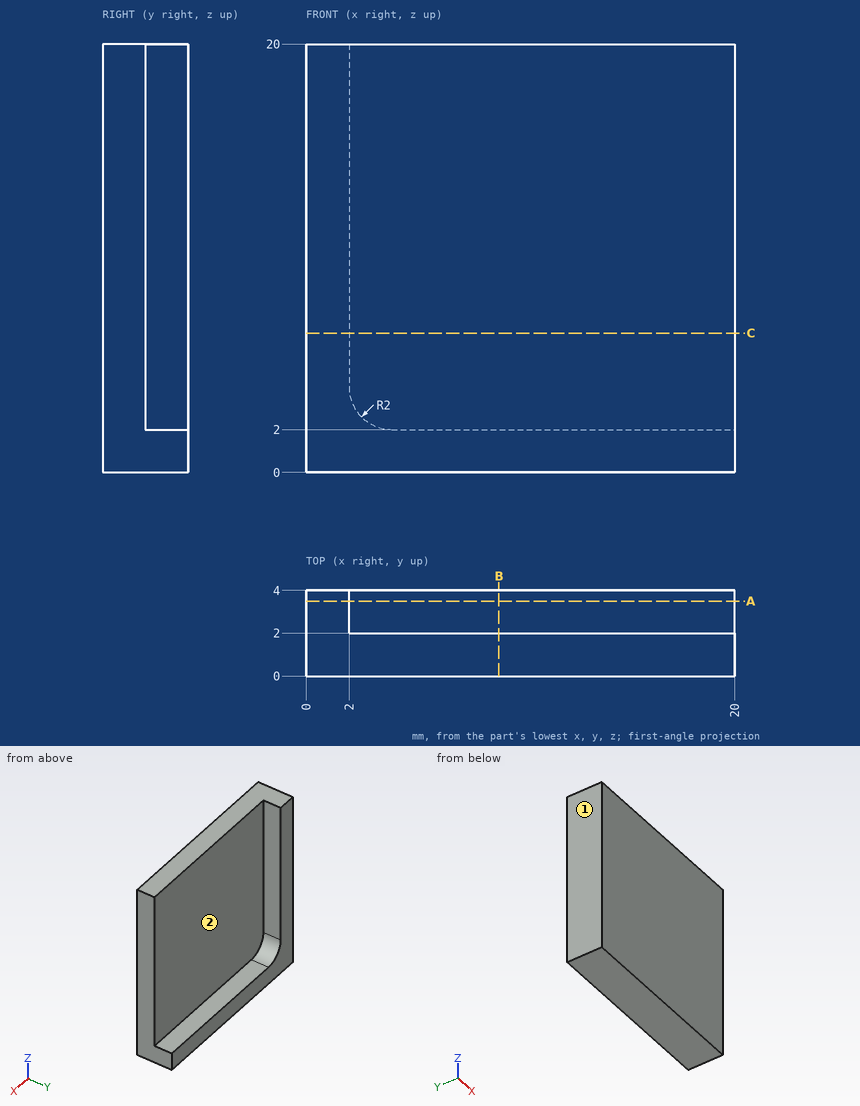
Can you work these out from the drawing? Everything is in mm from the part's minimum corner. A direction names the side the tool comes from. Round coordinates to 2 decimals unless told otherwise and drop trailing zeros. Loops run counter-clockwise (first coordinate to the right, second up) from the corner with the lowest first, then second, coordinate; pieces in that order, holes last. Notation, with made-up numbers: M -18.5,26 L -9.5,26 A16 cw -9.5,43 Z; hole C -31.75,45 d11. An arc over 180 degrees is marked long. Answer in a Markdown table with one row per item.
1. I'm going to push flat-ended pins straight in: pin 1 Ø10 at (x, z) = (5, 8) entering from +Y; pin 2 Ø8 at (x, z) = (7.5, 15.5) entering from +Y; pin 3 Ø1 at (y, z) = (3, 9.5) entering from +X; pin 4 Ø0.6 at (x, y) = (8.5, 3) entering from +Z. Where does each tip first touch, or does it pass through?
Established:
| item | result |
|---|---|
| pin 1 | y = 4 |
| pin 2 | y = 2 |
| pin 3 | x = 2 |
| pin 4 | z = 2 |
2. Please list where this line runs through material, in increasing order: line 1 (Y direction, x = 16, z = 5). Write a range as from..to.
Established:
| item | result |
|---|---|
| line 1 | 0..2 |
3. If we section it at C-C, the plane z = 6.5: Please give me the cut outline in (x, y).
Established:
| item | result |
|---|---|
| outline | M 0,0 L 20,0 L 20,2 L 2,2 L 2,4 L 0,4 Z |
4. If we section it at B-B, the plane x = 9: Please give me the cut outline in (y, z).
Established:
| item | result |
|---|---|
| outline | M 0,0 L 4,0 L 4,2 L 2,2 L 2,20 L 0,20 Z |
5. If we section it at A-A, the plane y = 3.5: Please give me the cut outline in (x, z), plus the area to 3 significant figures.
Established:
| item | result |
|---|---|
| outline | M 0,0 L 20,0 L 20,2 L 4,2 A2 cw 2,4 L 2,20 L 0,20 Z |
| area | 76.9 mm² |
6. On a 3-axis mill with a long thin cutter (end or side, diameter ignored), from which of +Z, -Z, +X, -X, +Y, -Y can I reach the whole of each face in a straight line? I mean the marked faces 1 and 2. Say none if no direction works.
Established:
| item | result |
|---|---|
| face 1 | +Z, -Z, -X, +Y, -Y |
| face 2 | +Z, +X, +Y |
